Verification items for the finished model (mm, model axes). Face numbers are marked on the shaded views. A direction names the side the tool comes from. Give positions to 0.01 mm unless a question says otherwise; leave off trailing zeros. Write each loop counter-clockwise with the first axis right and the second up, starting at its lowest first coordinate (ties: lowest second). Pieces come first, ordered by that corner, then holes. Notation, with made-up numbers: (62, 79) -> (67, 79) arc R14 cw to (67, 99) -> close; hole circle Ø1 at (-0.5, 31.5). An arc over 180 degrees is marked (long way). Use one line per item in the form item = value. Start each with the question number.
(1) Section check A-A, the plane y = 1.25. Record the cut outline in (x, z).
(2) Set-up check for the marked faces 5 and 6: record each of +Z, -Z, +X, -X, +Y, -Y from which the full face is reachable in a straight line by a thin tool's end or side.
(3) Section check D-D, the plane y = 8.75. Record the cut outline in (x, z).
(4) Section check C-C, the plane x = 11.9. Record the cut outline in (y, z).
(5) Scan lines: L1, parallel to X at y = 5.25, z = -7.9; L2, parallel to X at y = 9, z = -3.25; L3, parallel to Z at x = 7.5, y = 6. Record each from-to range of solid material in increasing order.
(6) Release check for a two-part mould opening along X. For the marked faces 1, 2, 3 and 4 record: pulls with the +X half, pulls with the -X half, needs draft (parallel to the pull), parting line crosses it, or undercut.
(7) Depth check by flat-ended pin: pin 1 Ø2.5 at (x, z) = (20.5, -11.5) entering from -Y; pin 2 Ø1.2 at (x, z) = (12, -12) entering from -Y; pin 3 Ø6.5 at (x, z) = (12, -5.5) entering from -Y. Enter the tip coordinate at first touch or a pass-through.
(8) Section check B-B, the plane z = -7.9. Record the cut outline in (x, y).
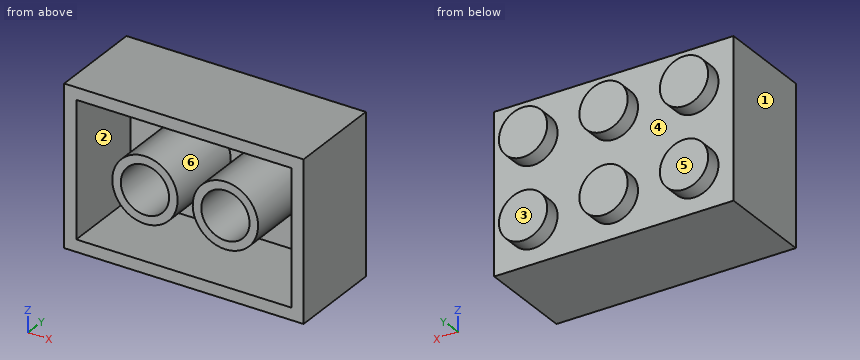
from build123d import *

# Parameters (mm, degrees)
SKETCH1_W            = 23.8
SKETCH1_H            = 9.6
BOSS_EXTRUDE1_DEPTH  = 15.8
SKETCH2_R            = 2.4
BOSS_EXTRUDE2_DEPTH  = 1.6
LPATTERN1_COUNT      = 3
LPATTERN1_PITCH      = 8
LPATTERN1_COUNT_DIR2 = 2
LPATTERN1_PITCH_DIR2 = 8
SHELL1_T             = -1.2
SKETCH3_R            = 3.25
SKETCH3_R_2          = 2.4
BOSS_EXTRUDE3_DEPTH  = 8.2
LPATTERN2_COUNT      = 2
LPATTERN2_PITCH      = 8


with BuildPart() as part:
    # Sketch1 → Boss-Extrude1 (new body)
    with BuildSketch(Plane.XY):
        with Locations((11.9, 4.8)):
            Rectangle(SKETCH1_W, SKETCH1_H)
    extrude(amount=-BOSS_EXTRUDE1_DEPTH)

    # Sketch2 → Boss-Extrude2 (add)
    with BuildSketch(Plane(origin=(0, 9.6, 0), x_dir=(1, 0, 0), z_dir=(0, 1, 0))):
        with Locations(Location((3.9, 3.9, 0), (0, 0, 90))):
            Circle(SKETCH2_R)
    boss_extrude2 = extrude(amount=BOSS_EXTRUDE2_DEPTH)

    # LPattern1: Boss-Extrude2 3 × 2
    with Locations(*[(i * LPATTERN1_PITCH, 0, -j * LPATTERN1_PITCH_DIR2) for i in range(LPATTERN1_COUNT) for j in range(LPATTERN1_COUNT_DIR2) if (i, j) != (0, 0)]):
        add(boss_extrude2)

    # Shell1
    shell1_openings = [part.faces().sort_by_distance(p)[0] for p in [
        (11.9, 0, -7.9),
    ]]
    offset(amount=SHELL1_T, openings=shell1_openings, kind=Kind.INTERSECTION)

    # Sketch3 → Boss-Extrude3 (add)
    with BuildSketch(Plane.XZ.offset(-8.4)):
        with Locations(Location((7.9, -7.9, 0), (0, 0, 270))):
            Circle(SKETCH3_R)
        with Locations(Location((7.9, -7.9, 0), (0, 0, 270))):
            Circle(SKETCH3_R_2, mode=Mode.SUBTRACT)
    boss_extrude3 = extrude(amount=BOSS_EXTRUDE3_DEPTH)

    # LPattern2: Boss-Extrude3 ×2
    with Locations(*[(i * LPATTERN2_PITCH, 0, 0) for i in range(1, LPATTERN2_COUNT)]):
        add(boss_extrude3)


solid = part.part
Completed:
q1.outline = (0, -15.8) -> (23.8, -15.8) -> (23.8, 0) -> (0, 0) -> close; circle Ø6.5 at (7.9, -7.9); circle Ø6.5 at (15.9, -7.9); hole (1.2, -14.6) -> (22.6, -14.6) -> (22.6, -1.2) -> (1.2, -1.2) -> close; hole circle Ø4.8 at (7.9, -7.9); hole circle Ø4.8 at (15.9, -7.9)
q2.face_5 = +Z, -Z, +X, -X, +Y
q2.face_6 = -Y
q3.outline = (0, -15.8) -> (23.8, -15.8) -> (23.8, 0) -> (0, 0) -> close; hole circle Ø2.4 at (3.9, -11.9); hole circle Ø2.4 at (3.9, -3.9); hole circle Ø2.4 at (11.9, -11.9); hole circle Ø2.4 at (11.9, -3.9); hole circle Ø2.4 at (19.9, -11.9); hole circle Ø2.4 at (19.9, -3.9)
q4.outline = (0, -15.8) -> (9.6, -15.8) -> (9.6, -14.3) -> (11.2, -14.3) -> (11.2, -9.5) -> (9.6, -9.5) -> (9.6, -6.3) -> (11.2, -6.3) -> (11.2, -1.5) -> (9.6, -1.5) -> (9.6, 0) -> (0, 0) -> (0, -1.2) -> (8.4, -1.2) -> (8.4, -2.7) -> (10, -2.7) -> (10, -5.1) -> (8.4, -5.1) -> (8.4, -10.7) -> (10, -10.7) -> (10, -13.1) -> (8.4, -13.1) -> (8.4, -14.6) -> (0, -14.6) -> close
q5.L1 = 0 to 1.2, 4.65 to 5.5, 10.3 to 11.15, 12.65 to 13.5, 18.3 to 19.15, 22.6 to 23.8
q5.L2 = 0 to 2.89, 4.91 to 10.89, 12.91 to 18.89, 20.91 to 23.8
q5.L3 = -15.8 to -14.6, -11.13 to -10.27, -5.53 to -4.67, -1.2 to 0
q6.face_1 = pulls with the -X half
q6.face_2 = undercut
q6.face_3 = needs draft
q6.face_4 = undercut
q7.pin_1 = 8.4
q7.pin_2 = 10
q7.pin_3 = 0.2
q8.outline = (0, 0) -> (1.2, 0) -> (1.2, 8.4) -> (4.65, 8.4) -> (4.65, 0.2) -> (5.5, 0.2) -> (5.5, 8.4) -> (10.3, 8.4) -> (10.3, 0.2) -> (11.15, 0.2) -> (11.15, 8.4) -> (12.65, 8.4) -> (12.65, 0.2) -> (13.5, 0.2) -> (13.5, 8.4) -> (18.3, 8.4) -> (18.3, 0.2) -> (19.15, 0.2) -> (19.15, 8.4) -> (22.6, 8.4) -> (22.6, 0) -> (23.8, 0) -> (23.8, 9.6) -> (0, 9.6) -> close
